Can you work these out from the model? Positions are in its coordinate system, mm. Round coordinates to 2 decimals unless told otherwise and drop trailing zeros. Loops run counter-clockwise (first coordinate to the right, second up) from the corner with the lowest first, then second, coordinate; pieces in that order, holes last.
(1) I want a section at B-B on x = 7. Write out the boundary of the cut face in (y, z), plus the area to 3 significant figures.
(2) If I drill on line 1 along Z through (x, y) = (7, 5.5); line 2 along X through (y, z) = (3, 9); line 3 along X through (y, z) = (0.5, 27), over which ranges is the centre line in solid material (lowest first)?
(3) I want a section at A-A on y = 0.5. Write out the boundary of the cut face in (x, z), plus the area to 3 significant figures.
(4) I want a section at C-C on z = 27. Write out the boundary of the cut face in (x, y).
(5) Will these pins go through, and if not, where does the flat tip stop? pin 1 Ø1 at (x, z) = (-4, 6) entering from +Y; pin 2 Ø4.5 at (x, z) = (7, 27) entering from +Y; pin 3 Ø1.5 at (y, z) = (-9.5, 10.5) entering from -X.
(6) I want a section at D-D on y = 5. Write out the boundary of the cut face in (x, z), plus the area to 3 significant figures.
(7) Thinking about a two-plate mould opening in X: for faces 1 (the face through (-12.488, 0.55, 17.748)), 2 (the face through (5, 0, 9)), 3 (the face through (-0.867, -3.905, 18.252)), 4 (the face through (-3, 3, 36)), which applies, released by +X, released by -X, zero draft, split by the parting line, or undercut?
from build123d import *

# Parameters (mm, degrees)
SKETCH_1_R               = 12.5
EXTRUDE_1_DEPTH          = 36
SKETCH_3_R               = 4
CUT_EXTRUDE_1_DEPTH      = 41.10610926
CUT_EXTRUDE_2_DEPTH      = 41.10610926
CUT_EXTRUDE_2_DEPTH_BACK = 41.10610926
SKETCH_4_R               = 2


with BuildPart() as part:
    # 草图1 → 拉伸1 (new body)
    with BuildSketch(Plane.XY):
        Circle(SKETCH_1_R)
    extrude(amount=EXTRUDE_1_DEPTH)

    # 草图3 → 切除-拉伸1 (cut, through all)
    with BuildSketch(Plane.XY.offset(36)):
        Circle(SKETCH_3_R)
    extrude(amount=-CUT_EXTRUDE_1_DEPTH, mode=Mode.SUBTRACT)

    # 草图4 → 切除-拉伸2 (cut, two sides: drawn at the far end of the back side and taken through both)
    with BuildSketch(Plane(origin=(0, 0, 0), x_dir=(1, 0, 0), z_dir=(0, 1, 0)).offset(-CUT_EXTRUDE_2_DEPTH_BACK)):
        with Locations(Location((7, -9, 0), (0, 0, 270))):
            Circle(SKETCH_4_R)
        with Locations(Location((7, -27, 0), (0, 0, 270))):
            Circle(SKETCH_4_R)
    extrude(amount=CUT_EXTRUDE_2_DEPTH + CUT_EXTRUDE_2_DEPTH_BACK, mode=Mode.SUBTRACT)


solid = part.part
Filled sheet:
1. outline: (-10.36, 0) - (10.36, 0) - (10.36, 7) - (-10.36, 7) - close; (-10.36, 11) - (10.36, 11) - (10.36, 25) - (-10.36, 25) - close; (-10.36, 29) - (10.36, 29) - (10.36, 36) - (-10.36, 36) - close
1. area: 580 mm2
2. line 1: z = 0 to 7, 11 to 25, 29 to 36
2. line 2: x = -12.13 to -2.65, 2.65 to 5, 9 to 12.13
2. line 3: x = -12.49 to -3.97, 3.97 to 5, 9 to 12.49
3. outline: (-12.49, 0) - (-3.97, 0) - (-3.97, 36) - (-12.49, 36) - close; (3.97, 0) - (12.49, 0) - (12.49, 36) - (3.97, 36) - close; hole circle Ø4 at (7, 9); hole circle Ø4 at (7, 27)
3. area: 588 mm2
4. outline: (5, -11.46) - (5, 11.46) arc R12.5 ccw (long way) to start; (9, -8.67) arc R12.5 ccw to (9, 8.67) - close; hole circle Ø8 at (0, 0)
5. pin 1: stops at y = 12
5. pin 2: stops at y = 11.56
5. pin 3: stops at x = -8.93
6. outline: (-11.46, 0) - (11.46, 0) - (11.46, 36) - (-11.46, 36) - close; hole circle Ø4 at (7, 9); hole circle Ø4 at (7, 27)
6. area: 800 mm2
7. face 1: split by the parting line
7. face 2: undercut
7. face 3: undercut
7. face 4: zero draft
